The model under review builds one solid part; all positions refer to its coordinate system, in mm. A direction names the side the tool comes from. Coordinates: 2 decimals unless noted, no trailing zeros. Write each loop counter-clockwise with the first axis right and the second up, starting at its lowest first coordinate (ties: lowest second). Pieces come first, ordered by that corner, then holes. Notation, with made-up numbers: (59.25, 4) -> (75.25, 4) arc R22 ccw to (75.25, 10) -> close; hole circle Ø9 at (-40, 83.25). An arc over 180 degrees is marked (long way). Write each question's results on one line, items separated by ' | '.
```python
from build123d import *

# Parameters (mm, degrees)
BOSS_EXTRUDE1_DEPTH                             = 30
BOSS_EXTRUDE2_DEPTH                             = 43.2
CSK_FOR_M5_FLAT_HEAD_MACHINE_SCREW1_D           = 5.5
CSK_FOR_M5_FLAT_HEAD_MACHINE_SCREW1_CSINK_D     = 10.4
CSK_FOR_M5_FLAT_HEAD_MACHINE_SCREW1_CSINK_ANGLE = 90
CSK_FOR_M5_FLAT_HEAD_MACHINE_SCREW2_D           = 5.5
CSK_FOR_M5_FLAT_HEAD_MACHINE_SCREW2_CSINK_D     = 10.4
CSK_FOR_M5_FLAT_HEAD_MACHINE_SCREW2_CSINK_ANGLE = 90
CUT_EXTRUDE1_DEPTH                              = 10
FILLET3_R                                       = 20
FILLET4_R                                       = 5


with BuildPart() as part:
    # Sketch1 → Boss-Extrude1 (new body)
    with BuildSketch(Plane(origin=(0, 0, 0), x_dir=(1, 0, 0), z_dir=(0, 1, 0))):
        Polygon((20, 20), (0, 0), (40, 0), (40, 20), align=None)
        Polygon((40, 0), (0, 0), (-30, -30), (40, -30), align=None)
    extrude(amount=-BOSS_EXTRUDE1_DEPTH)

    # Sketch1<3> → Boss-Extrude2 (add)
    with BuildSketch(Plane(origin=(0, 0, 0), x_dir=(1, 0, 0), z_dir=(0, 1, 0))):
        Polygon((40, 0), (0, 0), (-30, -30), (40, -30), align=None)
    extrude(amount=BOSS_EXTRUDE2_DEPTH)

    # CSK for M5 Flat Head Machine Screw1 (through all)
    with Locations(Plane.XY.offset(30)):
        with Locations((30, 10)):
            CounterSinkHole(CSK_FOR_M5_FLAT_HEAD_MACHINE_SCREW1_D / 2, CSK_FOR_M5_FLAT_HEAD_MACHINE_SCREW1_CSINK_D / 2, counter_sink_angle=CSK_FOR_M5_FLAT_HEAD_MACHINE_SCREW1_CSINK_ANGLE)

    # CSK for M5 Flat Head Machine Screw2 (through all)
    with Locations(Plane(origin=(0, -30, 0), x_dir=(-1, 0, 0), z_dir=(0, -1, 0))):
        with Locations((-30, 10)):
            CounterSinkHole(CSK_FOR_M5_FLAT_HEAD_MACHINE_SCREW2_D / 2, CSK_FOR_M5_FLAT_HEAD_MACHINE_SCREW2_CSINK_D / 2, counter_sink_angle=CSK_FOR_M5_FLAT_HEAD_MACHINE_SCREW2_CSINK_ANGLE)

    # Sketch10 → Cut-Extrude1 (cut)
    with BuildSketch(Plane(origin=(0, 43.2, 0), x_dir=(1, 0, 0), z_dir=(0, 1, 0))):
        Polygon((0, 0), (-1, -1), (40, -1), (40, 0), align=None)
    extrude(amount=-CUT_EXTRUDE1_DEPTH, mode=Mode.SUBTRACT)

    # Mirror2: part across plane


with BuildPart() as part_1:
    add(part.part)
    add(part.part.mirror(Plane(origin=(0, -30, 0), x_dir=(-0.7071067811865513, 0, 0.7071067811865438), z_dir=(-0.7071067811865439, 0, -0.7071067811865512))))

    # Fillet3
    fillet3_edges = [part_1.edges().sort_by_distance(p)[0] for p in [
        (5, -30, 30),
        (-30, 6.6, 30),
        (-30, -30, -5),
    ]]
    fillet(fillet3_edges, radius=FILLET3_R)

    # Fillet4
    # the kernel refuses this fillet: 5 mm, written as the material it adds along each edge
    with BuildSketch(Plane(origin=(20, 0, -20), x_dir=(1, 0, 0), z_dir=(0, -1, 0))) as fillet4_piece_1:
        with BuildLine():
            CenterArc((FILLET4_R, -FILLET4_R), FILLET4_R, 90, 90)
            Line((0, -FILLET4_R), (0, 0))
            Line((0, 0), (FILLET4_R, 0))
        make_face()
    extrude(amount=30)
    # the kernel refuses this fillet: 5 mm, written as the material it takes off along each edge
    with BuildSketch(Plane(origin=(40, -10, 30), x_dir=(0, 0, -1), z_dir=(0, 1, 0))) as fillet4_2_piece_1:
        with BuildLine():
            CenterArc((FILLET4_R, FILLET4_R), FILLET4_R, 180, 90)
            Line((0, FILLET4_R), (0, 0))
            Line((0, 0), (FILLET4_R, 0))
        make_face()
    extrude(amount=65.7, mode=Mode.SUBTRACT)
    with BuildSketch(Plane(origin=(40, -30, -32.5), x_dir=(0, 1, 0), z_dir=(0, 0, 1)), Plane(origin=(32.5, -30, -40), x_dir=(0, 0, 1), z_dir=(-1, 0, 0))) as fillet4_2_piece_2:
        with BuildLine():
            CenterArc((FILLET4_R, FILLET4_R), FILLET4_R, 180, 90)
            Line((0, FILLET4_R), (0, 0))
            Line((0, 0), (FILLET4_R, 0))
        make_face()
    extrude(amount=42.5, mode=Mode.SUBTRACT)
    with BuildSketch(Plane(origin=(40, -10, 10), x_dir=(0, -1, 0), z_dir=(0, 0, -1))) as fillet4_2_piece_3:
        with BuildLine():
            CenterArc((20 - FILLET4_R, FILLET4_R), FILLET4_R, 270, 90)
            Line((20, FILLET4_R), (20, 0))
            Line((20, 0), (20 - FILLET4_R, 0))
        make_face()
    revolve(axis=Axis((40, -10, 10), (-1, 0, 0)), revolution_arc=90, mode=Mode.SUBTRACT)
    with BuildSketch(Plane(origin=(-30, -10, -40), x_dir=(1, 0, 0), z_dir=(0, 1, 0))) as fillet4_2_piece_4:
        with BuildLine():
            CenterArc((FILLET4_R, -FILLET4_R), FILLET4_R, 90, 90)
            Line((0, -FILLET4_R), (0, 0))
            Line((0, 0), (FILLET4_R, 0))
        make_face()
    extrude(amount=65.7, mode=Mode.SUBTRACT)
    with BuildSketch(Plane(origin=(-10, -10, -40), x_dir=(0, -1, 0), z_dir=(1, 0, 0))) as fillet4_2_piece_5:
        with BuildLine():
            CenterArc((20 - FILLET4_R, -FILLET4_R), FILLET4_R, 0, 90)
            Line((20 - FILLET4_R, 0), (20, 0))
            Line((20, 0), (20, -FILLET4_R))
        make_face()
    revolve(axis=Axis((-10, -10, -40), (0, 0, -1)), revolution_arc=90, mode=Mode.SUBTRACT)


solid = part_1.part
```
Q1. Add section C-C (y = -7.5). Write out the cut boundary in (x, z).
Solution:
outline: (-30, -35) arc R5 ccw to (-25, -40) -> (20, -40) -> (20, -25) arc R5 cw to (25, -20) -> (40, -20) -> (40, 25) arc R5 ccw to (35, 30) -> (-10, 30) arc R20 ccw to (-30, 10) -> close; hole circle Ø5.5 at (10, -30); hole circle Ø5.5 at (30, -10)
Q2. For line 1 (Z direction, x = -6, y = 10); line 2 (Y direction, x = 30, z = 8.75); line 3 (Y direction, x = 22, z = -15.5), list the stretches that pass through material, from the lowest coordinate up. Write a range as from..to.
Solution:
line 1: -40..-32.75, -27.25..30 | line 2: -30..7.25, 12.75..43.2 | line 3: -30..0
Q3. Add section D-D (z = -10). Write out the cut boundary in (x, y).
Solution:
outline: (-30, -10) arc R20 ccw to (-10, -30) -> (24.8, -30) -> (27.25, -27.55) -> (27.25, 0) -> (0, 0) -> (0, 33.2) -> (-1, 33.2) -> (-1, 43.2) -> (-30, 43.2) -> close; (32.75, -27.55) -> (35.2, -30) arc R5 ccw to (40, -25) -> (40, 0) -> (32.75, 0) -> close
Q4. Machinability: for faces 1 (the flat face through (-2, 43.2, 3)), 2 (the flat face through (16, 0, -15)), which of the approach directions +Z, -Z, +X, -X, +Y, -Y give a long, thin tool a straight path to every point of the face, cutting with its end or side? Answer none if there is none.
Solution:
face 1: +Z, -Z, +X, -X, +Y | face 2: -Z, +X, +Y
Q5. Add section B-B (x = 30). Write out the cut boundary in (y, z), plus the area to 3 significant figures.
Solution:
outline: (-30, -20) -> (0, -20) -> (0, -12.75) -> (-27.55, -12.75) -> (-30, -15.2) -> close; (-30, -4.8) -> (-27.55, -7.25) -> (0, -7.25) -> (0, 0) -> (7.25, 0) -> (7.25, 27.55) -> (4.8, 30) -> (-10, 30) arc R20 ccw to (-30, 10) -> close; (12.75, 0) -> (33.2, 0) -> (33.2, 1) -> (43.2, 1) -> (43.2, 30) -> (15.2, 30) -> (12.75, 27.55) -> close | area: 2,360 mm²
Q6. Clearance check with flat-ended pins moving along their axes: P1, Ø1.5, axis at y = 33, z = -25.5, coming from the +X side; P2, Ø3.5, axis at y = 10, z = -30, coming from the -X side; P3, Ø4.5, axis at x = 33, y = -16.5, coming from the -Z side; P4, Ø6.5, axis at x = 30, z = -10, coming from the -Y side. State where each tip first meets the part, or that it passes through.
Solution:
P1: x = 0 | P2: through | P3: z = -20 | P4: y = -28.05
Q7. Add section A-A (z = -30). Write out the cut boundary in (x, y), plus the area to 3 significant figures.
Solution:
outline: (-30, -10) arc R20 ccw to (-10, -30) -> (4.8, -30) -> (7.25, -27.55) -> (7.25, 0) -> (0, 0) -> (0, 7.25) -> (-27.55, 7.25) -> (-30, 4.8) -> close; (-30, 15.2) -> (-27.55, 12.75) -> (0, 12.75) -> (0, 33.2) -> (-1, 33.2) -> (-1, 43.2) -> (-30, 43.2) -> close; (12.75, -27.55) -> (15.2, -30) -> (20, -30) -> (20, 0) -> (12.75, 0) -> close | area: 2,360 mm²
Q8. Draft analysis for pull direction Z (two halves, no side actions). For faces 3 (the cylindrical face through (27.253, -13.582, -10.121)), 4 (the flat face through (12, 16, 30)), 5 (the cylindrical face through (22, -15, -21)), state which applies: pulls with the +Z half, pulls with the -Z half, needs draft (parallel to the pull), parting line crosses it, or undercut.
Solution:
face 3: undercut | face 4: pulls with the +Z half | face 5: pulls with the -Z half
